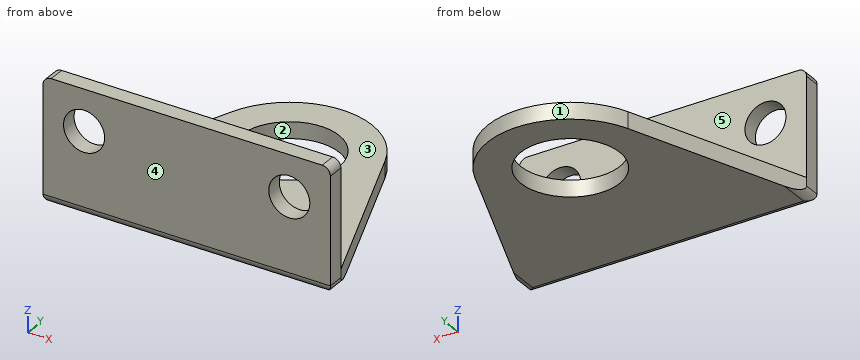
```python
from build123d import *

# Parameters (mm, degrees)
SKETCH1_W           = 35
SKETCH1_H           = 15
BOSS_EXTRUDE1_DEPTH = 2
BOSS_EXTRUDE2_DEPTH = 2
FILLET1_R           = 10
FILLET2_R           = 1
FILLET3_R           = 1
SKETCH4_R           = 2.5
CUT_EXTRUDE1_DEPTH  = 3
SKETCH5_R           = 6
CUT_EXTRUDE2_DEPTH  = 3


with BuildPart() as part:
    # Sketch1 → Boss-Extrude1 (new body)
    with BuildSketch(Plane(origin=(0, 0, 0), x_dir=(1, 0, 0), z_dir=(0, 1, 0))):
        with Locations((17.5, 7.5)):
            Rectangle(SKETCH1_W, SKETCH1_H)
    extrude(amount=BOSS_EXTRUDE1_DEPTH)

    # Sketch3 → Boss-Extrude2 (add)
    with BuildSketch(Plane(origin=(0, 0, -15), x_dir=(-1, 0, 0), z_dir=(0, 0, -1))):
        Polygon((0, 2), (-35, 2), (-17.5, 47.5), align=None)
    extrude(amount=-BOSS_EXTRUDE2_DEPTH)

    # Fillet1
    fillet1_edges = [part.edges().sort_by_distance(p)[0] for p in [
        (17.5, 47.5, -14),
    ]]
    fillet(fillet1_edges, radius=FILLET1_R)

    # Fillet2
    fillet2_edges = [part.edges().sort_by_distance(p)[0] for p in [
        (17.5, 0, -15),
        (0, 1, -15),
        (35, 1, -15),
    ]]
    fillet(fillet2_edges, radius=FILLET2_R)

    # Fillet3
    fillet3_edges = [part.edges().sort_by_distance(p)[0] for p in [
        (35, 1, 0),
        (0, 1, 0),
    ]]
    fillet(fillet3_edges, radius=FILLET3_R)

    # Sketch4 → Cut-Extrude1 (cut, through all)
    with BuildSketch(Plane(origin=(0, 2, 0), x_dir=(1, 0, 0), z_dir=(0, 1, 0))):
        with Locations((5, 5)):
            Circle(SKETCH4_R)
        with Locations((30, 5)):
            Circle(SKETCH4_R)
    extrude(amount=-CUT_EXTRUDE1_DEPTH, mode=Mode.SUBTRACT)

    # Sketch5 → Cut-Extrude2 (cut, through all)
    with BuildSketch(Plane.XY.offset(-13)):
        with Locations((17.5, 19.643223446)):
            Circle(SKETCH5_R)
    extrude(amount=-CUT_EXTRUDE2_DEPTH, mode=Mode.SUBTRACT)


solid = part.part
```
Can you work these out from the model? Positions are in its coordinate system, mm. Face numbers are marked on the shaded views. A direction names the side the tool comes from. Coordinates: 2 decimals unless noted, no trailing zeros. Order: outer loops, then holes, each group sorted by start corner. A loop starts at its lowest first (then second) coordinate and runs counter-clockwise, first axis right, second up.
1. I'm going to push flat-ended pins straight in: pin 1 (4 mm diameter, centred on x = 20, z = -9.5, fed in from +Y); pin 2 (5 mm diameter, centred on x = 19.5, y = 15, fed in from +Z); pin 3 (11 mm diameter, centred on x = 17.5, y = 19.64, fed in from +Z). Where does each tip first touch, or does it pass through?
2. If we section it at D-D (x = 30): Please give me the cut outline in (y, z).
3. If we section it at C-C (y = 21.5): Please give me the cut outline in (x, z), then the cut area to 3 significant figures.
4. Thinking about a two-plate mould opening in X: for the marked faces 1, 2 and 3, which applies, +X half, -X half, draft (parallel to the pull), parting line (faces both ways), or undercut?
5. For the marked faces 4 and 5, which set-ups out of +Z, -Z, +X, -X, +Y, -Y let a thin tool reach every point of the face, with its end or its side?
6. If we section it at B-B (z = -5): Please give me the cut outline in (x, y).
7. If we section it at A-A (x = 17.5): Please give me the cut outline in (y, z), then the cut area to 3 significant figures.
8. I need wall thicknesses on line 1 (X direction, y = 1.4, z = -5); line 2 (Y direction, x = 17.5, z = -14); line 3 (Z direction, x = 5, y = 0.95). Which ranges of each line are inside material? Lowest first, please.
Entries:
1. pin 1: stops at y = 2
1. pin 2: stops at z = -13
1. pin 3: passes through
2. outline: (0, -14) arc R1 ccw to (1, -15) - (15, -15) - (15, -13) - (2, -13) - (2, -7.5) - (0, -7.5) - close; (0, -2.5) - (2, -2.5) - (2, 0) - (0, 0) - close
3. outline: (7.5, -15) - (11.79, -15) - (11.79, -13) - (7.5, -13) - close; (23.21, -15) - (27.5, -15) - (27.5, -13) - (23.21, -13) - close
3. area: 17.2 mm2
4. face 1: parting line
4. face 2: undercut
4. face 3: draft
5. face 4: +Z, -Z, +X, -X, -Y
5. face 5: +Z, +X, -X, +Y
6. outline: (0, 0) - (2.5, 0) - (2.5, 2) - (0, 2) - close; (7.5, 0) - (27.5, 0) - (27.5, 2) - (7.5, 2) - close; (32.5, 0) - (35, 0) - (35, 2) - (32.5, 2) - close
7. outline: (0, -14) arc R1 ccw to (1, -15) - (13.64, -15) - (13.64, -13) - (2, -13) - (2, 0) - (0, 0) - close; (25.64, -15) - (29.64, -15) - (29.64, -13) - (25.64, -13) - close
7. area: 61.1 mm2
8. line 1: x = 0 to 2.5, 7.5 to 27.5, 32.5 to 35
8. line 2: y = 0 to 13.64, 25.64 to 29.64
8. line 3: z = -15 to -7.5, -2.5 to 0
